Autodesk Inventor part; units mm, degrees
ref_plane "YZ Plane" through (0, 0, 0) normal (1, 0, 0) x (0, 1, 0)
ref_plane "XZ Plane" through (0, 0, 0) normal (0, 1, 0) x (-1, 0, 0)
ref_plane "XY Plane" through (0, 0, 0) normal (0, 0, 1) x (1, 0, 0)
sketch "Эскиз1" plane through (0, 0, 0) normal (0, 1, 0) x (-1, 0, 0)
  circle A0 centre (-102.5556, 225.6292) radius 3.05
  circle A1 centre (-183.8617, 259.7302) radius 3.05
  circle A2 centre (-241.4187, 192.9413) radius 3.05
  circle A3 centre (-195.6847, 117.5625) radius 3.05
  circle A4 centre (-109.8626, 137.7647) radius 3.05
  line L0 (-177.5294, 108.3895) -> (-150.4825, 84.7228)
  arc A5 (-148.7964, 81.4219) -> (-142.475, 75.8905) centre (-142.7225, 81.9854) ccw
  line L1 (-138.9795, 74.6574) -> (-112.854, 51.7971)
  arc A6 (-111.168, 48.4962) -> (-98.9991, 49.3073) centre (-105.0941, 49.0597) ccw
  line L2 (-97.7661, 52.8028) -> (-70.8888, 83.5189)
  arc A7 (-67.5879, 85.2049) -> (-63.3144, 94.9954) centre (-68.1514, 91.2788) ccw
  line L3 (-63.3144, 94.9954) -> (-108.3131, 153.5599)
  arc A8 (-154.5301, 238.9315) -> (-170.0329, 240.2208) centre (-162.9261, 231.8247) ccw
  line L4 (-186.8375, 143.9878) -> (-185.285, 127.1516)
  arc A9 (-185.285, 127.1516) -> (-183.1128, 124.9467) centre (-183.2964, 126.9383) ccw
  line L5 (-183.1128, 124.9467) -> (-179.0904, 125.3176)
  line L6 (-179.0904, 125.3176) -> (-177.5294, 108.3895)
  circle A10 centre (-117.9158, 72.371) radius 3.05
  circle A11 centre (-155.5442, 105.2966) radius 3.05
  circle A12 centre (-130.5866, 133.819) radius 3.05
  circle A13 centre (-105.7799, 124.2045) radius 3.05
  circle A14 centre (-92.9581, 100.8933) radius 3.05
  circle A15 centre (-162.9261, 231.8247) radius 5.05
  circle A16 centre (-121.5775, 182.975) radius 5.05
  circle A17 centre (-105.0941, 49.0597) radius 3.05
  circle A18 centre (-142.7225, 81.9854) radius 3.05
  circle A19 centre (-68.1514, 91.2788) radius 3.05
  line L7 (-182.2769, 125.0238) -> (-180.8753, 109.8244)
  arc A20 (-179.9058, 262.7882) -> (-188.7663, 260.7024) centre (-183.8617, 259.7302) ccw
  arc A21 (-98.4249, 222.8119) -> (-103.1466, 230.5942) centre (-102.5556, 225.6292) ccw
  arc A22 (-200.6825, 117.4137) -> (-196.2371, 112.5931) centre (-195.6847, 117.5625) ccw
  arc A23 (-243.1045, 197.6485) -> (-243.8589, 188.5772) centre (-241.4187, 192.9413) ccw
  line L8 (-180.8753, 109.8244) -> (-196.5681, 112.6411)
  circle A24 centre (-166.6767, 186.7256) radius 85 construction
  line L9 (-99.8729, 142.5753) -> (-63.3144, 94.9954)
  arc A25 (-104.963, 159.8791) -> (-99.8729, 142.5753) centre (-80.049, 157.8072) ccw
  line L10 (-196.2294, 112.5804) -> (-196.2371, 112.5931)
  line L11 (-202.1286, 122.3034) -> (-240.1899, 185.0362)
  line L12 (-100.129, 218.0061) -> (-104.963, 159.8791)
  line L13 (-175.8619, 259.6823) -> (-108.1962, 231.3023)
  line L14 (-77.9802, 218.6293) -> (-73.529, 216.7624)
  arc A26 (-98.4249, 222.8119) -> (-100.129, 218.0061) centre (-90.1634, 217.1773) ccw
  arc A27 (-108.1962, 231.3023) -> (-103.1466, 230.5942) centre (-104.3284, 240.5241) ccw
  arc A28 (-179.9058, 262.7882) -> (-175.8619, 259.6823) centre (-171.9941, 268.9041) ccw
  arc A29 (-191.0002, 256.1188) -> (-188.7663, 260.7024) centre (-198.5754, 262.6469) ccw
  arc A30 (-243.1045, 197.6485) -> (-238.901, 200.5348) centre (-246.4763, 207.0629) ccw
  arc A31 (-240.1899, 185.0362) -> (-243.8589, 188.5772) centre (-248.7394, 179.8491) ccw
  arc A32 (-200.6825, 117.4137) -> (-202.1286, 122.3034) centre (-210.6781, 117.1163) ccw
  arc A33 (-148.7964, 81.4219) -> (-150.4825, 84.7228) centre (-153.775, 80.9599) ccw
  arc A34 (-138.9795, 74.6574) -> (-142.475, 75.8905) centre (-142.272, 70.8946) ccw
  arc A35 (-111.168, 48.4962) -> (-112.854, 51.7971) centre (-116.1466, 48.0342) ccw
  arc A36 (-97.7661, 52.8028) -> (-98.9991, 49.3073) centre (-94.0032, 49.5102) ccw
  arc A37 (-67.5879, 85.2049) -> (-70.8888, 83.5189) centre (-67.1259, 80.2263) ccw
  arc A38 (-173.2989, 194.5492) -> (-160.0544, 178.902) centre (-166.6767, 186.7256) ccw
  arc A39 (-111.4672, 178.6413) -> (-108.3131, 153.5599) centre (-88.4892, 168.7918) ccw
  arc A40 (-111.4672, 178.6413) -> (-113.1815, 190.0818) centre (-121.5775, 182.975) ccw
  line L15 (-113.1815, 190.0818) -> (-127.2335, 206.6831)
  line L16 (-127.2335, 206.6831) -> (-160.0544, 178.902)
  line L17 (-173.2989, 194.5492) -> (-140.478, 222.3303)
  line L18 (-140.478, 222.3303) -> (-154.5301, 238.9315)
  line L19 (-170.0329, 240.2208) -> (-188.2631, 224.7899)
  arc A41 (-218.8826, 198.8722) -> (-220.1719, 183.3693) centre (-211.7758, 190.4761) ccw
  line L20 (-220.1719, 183.3693) -> (-186.8375, 143.9878)
  circle A42 centre (-170.4272, 141.6264) radius 5.05
  circle A43 centre (-211.7758, 190.4761) radius 5.05
  arc A44 (-154.7115, 183.4245) -> (-167.956, 199.0717) centre (-161.3337, 191.2481) ccw
  line L21 (-220.9265, 180.3759) -> (-221.3765, 181.0768)
  line L22 (-190.4765, 248.7938) -> (-191.1373, 255.9597)
  line L23 (-193.663, 248.4999) -> (-194.0403, 252.5911)
  line L24 (-190.4765, 248.7938) -> (-193.663, 248.4999)
  line L25 (-238.901, 200.5348) -> (-194.0403, 252.5911)
  line L26 (-191.1373, 255.9597) -> (-191.0002, 256.1188)
  line L27 (-188.2631, 224.7899) -> (-187.4464, 215.9332)
  line L28 (-187.4464, 215.9332) -> (-190.6328, 215.6393)
  line L29 (-190.6328, 215.6393) -> (-191.244, 222.2668)
  line L30 (-191.244, 222.2668) -> (-218.8826, 198.8722)
  point P0 (0, 0)
  point P1 (-98.7723, 141.1427)
  point P2 (-176.2905, 107.3053)
  point P3 (-200.3475, 119.3677)
  point P4 (-241.9711, 187.9719)
  point P5 (-241.1427, 197.9337)
  point P6 (-179.0284, 261.0104)
  point P7 (-188.7586, 258.72)
  point P8 (-99.8445, 221.4281)
  point P9 (-105.0296, 229.9742)
  point P10 (-99.8729, 142.5753)
  point P11 (-236.553, 192.5367)
  dimension "d5" = 6.1
  dimension "d8" = 360
  dimension "d13" = 3.2
  dimension "d16" = 10
  dimension "d26" = 170
  dimension "d31" = 25
  dimension "d32" = 10
  dimension "d33" = 10
  dimension "d34" = 10
  dimension "d35" = 10
  dimension "d36" = 7
  dimension "d37" = 75
  dimension "d46" = 124
extrude "Выдавливание1" add sketch "Эскиз1" along normal blind 3 contours L6 L5 A9 L4 L20 A41 L30 L29 L28 L27 L19 A8 L18 L17 A38 L16 L15 A40 A39 L3 A7 A37 L2 A36 A6 A35 L1 A34 A5 A33 L0 | L7 L8 L10 A22 A32 L11 A31 A23 A30 L25 L23 L24 L22 L26 A29 A20 A28 L13 A27 A21 A26 L12 A25 L3 A39 A40 L15 L16 A44 L17 L18 A8 L19 L27 L28 L29 L30 A41 L20 L4 A9 L5 | L8 A22 L10
sketch "Эскиз2" plane through (0, 3, 0) normal (0, 1, 0) x (1, 0, 0)
  line L0 (63.3144, -94.9954) -> (99.8729, -142.5753)
  arc A0 (104.963, -159.8791) -> (99.8729, -142.5753) centre (80.049, -157.8072) ccw
  line L1 (104.963, -159.8791) -> (100.129, -218.0061)
  arc A1 (98.4249, -222.8119) -> (100.129, -218.0061) centre (90.1634, -217.1773) ccw
  arc A2 (98.4249, -222.8119) -> (103.1466, -230.5942) centre (102.5556, -225.6292) ccw
  arc A3 (108.1962, -231.3023) -> (103.1466, -230.5942) centre (104.3284, -240.5241) ccw
  line L2 (108.1962, -231.3023) -> (175.8619, -259.6823)
  arc A4 (179.9058, -262.7882) -> (175.8619, -259.6823) centre (171.9941, -268.9041) ccw
  arc A5 (179.9058, -262.7882) -> (188.7663, -260.7024) centre (183.8617, -259.7302) ccw
  arc A6 (191.0002, -256.1188) -> (188.7663, -260.7024) centre (198.5754, -262.6469) ccw
  line L3 (194.0403, -252.5911) -> (238.901, -200.5348)
  arc A7 (243.1045, -197.6485) -> (238.901, -200.5348) centre (246.4763, -207.0629) ccw
  arc A8 (243.1045, -197.6485) -> (243.8589, -188.5772) centre (241.4187, -192.9413) ccw
  arc A9 (240.1899, -185.0362) -> (243.8589, -188.5772) centre (248.7394, -179.8491) ccw
  line L4 (240.1899, -185.0362) -> (202.1286, -122.3034)
  arc A10 (200.6825, -117.4137) -> (202.1286, -122.3034) centre (210.6781, -117.1163) ccw
  arc A11 (200.6825, -117.4137) -> (196.5681, -112.6411) centre (195.6847, -117.5625) ccw
  line L5 (196.5681, -112.6411) -> (180.8753, -109.8244)
  line L6 (180.8753, -109.8244) -> (182.2769, -125.0238)
  line L7 (182.2769, -125.0238) -> (179.0904, -125.3176)
  line L8 (179.0904, -125.3176) -> (177.5294, -108.3895)
  line L9 (177.5294, -108.3895) -> (150.4825, -84.7228)
  arc A12 (148.7964, -81.4219) -> (150.4825, -84.7228) centre (153.775, -80.9599) ccw
  arc A13 (148.7964, -81.4219) -> (142.475, -75.8905) centre (142.7225, -81.9854) ccw
  arc A14 (138.9795, -74.6574) -> (142.475, -75.8905) centre (142.272, -70.8946) ccw
  line L10 (138.9795, -74.6574) -> (112.854, -51.7971)
  arc A15 (111.168, -48.4962) -> (112.854, -51.7971) centre (116.1466, -48.0342) ccw
  arc A16 (111.168, -48.4962) -> (98.9991, -49.3073) centre (105.0941, -49.0597) ccw
  arc A17 (97.7661, -52.8028) -> (98.9991, -49.3073) centre (94.0032, -49.5102) ccw
  line L11 (97.7661, -52.8028) -> (70.8888, -83.5189)
  arc A18 (67.5879, -85.2049) -> (70.8888, -83.5189) centre (67.1259, -80.2263) ccw
  arc A19 (67.5879, -85.2049) -> (63.3144, -94.9954) centre (68.1514, -91.2788) ccw
  circle A20 centre (109.8626, -137.7647) radius 3.05
  circle A21 centre (117.9158, -72.371) radius 3.05
  circle A22 centre (155.5442, -105.2966) radius 3.05
  circle A23 centre (105.7799, -124.2045) radius 3.05
  circle A24 centre (92.9581, -100.8933) radius 3.05
  circle A25 centre (162.9261, -231.8247) radius 5.05
  circle A26 centre (105.0941, -49.0597) radius 3.05
  circle A27 centre (142.7225, -81.9854) radius 3.05
  circle A28 centre (68.1514, -91.2788) radius 3.05
  circle A29 centre (130.5866, -133.819) radius 3.05
  circle A30 centre (195.6847, -117.5625) radius 3.05
  circle A31 centre (241.4187, -192.9413) radius 3.05
  circle A32 centre (183.8617, -259.7302) radius 3.05
  circle A33 centre (102.5556, -225.6292) radius 3.05
  line L12 (191.0002, -256.1188) -> (191.1373, -255.9597)
  line L13 (191.1373, -255.9597) -> (190.4765, -248.7938)
  line L14 (190.4765, -248.7938) -> (193.663, -248.4999)
  line L15 (193.663, -248.4999) -> (194.0403, -252.5911)
  point P0 (0, 0)
equation "\"d5\" = d_main_screw_holes"
equation "\"d2\" = thickness_steel"
equation "\"tolerance_plazma\" = 0.1"
equation "\"thickness_steel\" = 3"
equation "\"d_main_screw_holes\" = 6.1"
equation "\"thickness_profile_tibea\" = 3"
equation "\"hight_shaft_shift\" = 37"
equation "\"thickness_profile_femur\" = 3"
equation "\"width_shaft_shift\" = 35"
equation "\"width_flattened_surface\" = 12"
equation "\"d22\" = d_main_screw_holes"
equation "\"d23\" = d_main_screw_holes"
equation "\"d25\" = d_main_screw_holes"
properties part number "femur_motor_steel" material "Сталь"
Geometry check sheet. Reference: the model listing, model coordinates, mm. A direction names the side the tool comes from. Give positions to 0.01 mm unless a question says otherwise; leave off trailing zeros. Write each loop counter-clockwise with the first axis right and the second up, starting at its lowest first coordinate (ties: lowest second). Pieces come first, ordered by that corner, then holes. Notation, with made-up numbers: M 16.5,79.5 L 47.5,79.5 A20 cw 47.5,91.5 Z; hole C 66,55.5 d10. An arc over 180 degrees is marked long. One line per question, with ' | ' between items.
1. Gauge pin test, flat ends, axial feed: pin 1 (5.5 mm diameter, centred on x = 68.15, z = 91.28, fed in from +Y); pin 2 (1.5 mm diameter, centred on y = 1, z = 126, fed in from +X); pin 3 (1.5 mm diameter, centred on y = 2, z = 176.5, fed in from +X). Record the tip position at first contact, or that the pin passes through.
Ans:
pin 1: through | pin 2: x = 204.83 | pin 3: x = 235.47
2. Set-up check for faces 1 (the face through (166.648, 1.479, 228.412)), 2 (the face through (102.512, 1.479, 189.349)): record each of +Z, -Z, +X, -X, +Y, -Y from which the full face is reachable in a straight line by a thin tool's end or side.
Ans:
face 1: +Y, -Y | face 2: -X, +Y, -Y
3. Cross-section at A-A (x = 210). Enter the section's corners in (y, z), plus the area to 3 significant figures.
Ans:
outline: M 0,135.28 L 3,135.28 L 3,185.75 L 0,185.75 Z; M 0,195.2 L 3,195.2 L 3,234.07 L 0,234.07 Z | area: 268 mm2
4. Cross-section at B-B (y = 1.05). Count the separate pieces of the cut face and the enclosed holes in it, plus the area to 3 significant figures.
Ans:
separate pieces: 1 | enclosed holes: 18 | area: 19,700 mm2
5. Cross-section at D-D (x = 232.5). Enter the section's corners in (y, z), plus the area to 3 significant figures.
Ans:
outline: M 0,172.36 L 3,172.36 L 3,207.96 L 0,207.96 Z | area: 107 mm2
6. Mould release check, pull along X, two halves, no side actions. Record for faces 3 (the face through (104.557, 1.479, 42.983)), 4 (the face through (157.35, 1.48, 181.19)), 5 (the face through (164.195, 1.479, 96.722)): released by +X, released by -X, zero draft, split by the parting line, or undercut.
Ans:
face 3: split by the parting line | face 4: undercut | face 5: released by +X
7. Cross-section at C-C (z = 207.5). Enter the section's corners in (x, y).
Ans:
outline: M 101,0 L 232.9,0 L 232.9,3 L 101,3 Z
8. Scan lines: line 1 along X through (y, z) = (2.3, 193); line 2 along X through (y, z) = (1, 121.5); line 3 along X through (y, z) = (1.8, 191.5). Record each from-to range of solid material in increasing order. Write a range as from..to.
Ans:
line 1: 102.21..151.23, 174.78..207.4, 216.15..238.37, 244.47..246.42 | line 2: 83.68..104.37, 107.19..178.74, 181.95..201.69 | line 3: 102.33..151.09, 175.75..206.83, 216.72..238.73, 244.11..246.21
